Source: CAD feature listing. Evaluate the final solid. Frame: model axes, mm. Give positions to 0.01 mm unless a question says otherwise; leave off trailing zeros. Loops run counter-clockwise (first coordinate to the right, second up) from the corner with the lowest first, then second, coordinate; pieces in that order, holes last. Notation, with made-up numbers: (27, -37) -> (81, -37) arc R21 ccw to (81, -33) -> close; hole circle Ø7 at (53.25, 15). An arc over 180 degrees is marked (long way). Put each result on its own line as item: value.
```python
from build123d import *

# Parameters (mm, degrees)
ESBO_O1_W                  = 54
ESBO_O1_H                  = 15
RESSALTO_EXTRUS_O1_DEPTH   = 1.2
CORTE_EXTRUS_O1_DEPTH      = 5
CORTE_EXTRUS_O1_DEPTH_BACK = 1.2
ESBO_O2_R                  = 2


with BuildPart() as part:
    # Esboço1 → Ressalto-extrusão1 (new body)
    with BuildSketch(Plane.XY):
        Rectangle(ESBO_O1_W, ESBO_O1_H)
    extrude(amount=RESSALTO_EXTRUS_O1_DEPTH)

    # Esboço2 → Corte-extrusão1 (cut, two sides: drawn at the far end of the back side and taken through both)
    with BuildSketch(Plane.XY.offset(-CORTE_EXTRUS_O1_DEPTH_BACK)):
        with Locations(Location((-21.8, 0, 0), (0, 0, 180))):
            Circle(ESBO_O2_R)
        with Locations(Location((21.8, 0, 0), (0, 0, 180))):
            Circle(ESBO_O2_R)
    extrude(amount=CORTE_EXTRUS_O1_DEPTH + CORTE_EXTRUS_O1_DEPTH_BACK, mode=Mode.SUBTRACT)


solid = part.part
```
(1) Section C-C on z = 0.9. Return loops of the section in (x, y), then the cut area to 3 significant figures.
Calculated:
outline: (-27, -7.5) -> (27, -7.5) -> (27, 7.5) -> (-27, 7.5) -> close; hole circle Ø4 at (-21.8, 0); hole circle Ø4 at (21.8, 0)
area: 785 mm²
(2) Section A-A on x = 21.8. Return loops of the section in (y, z), then the cut area to 3 significant figures.
Calculated:
outline: (-7.5, 0) -> (-2, 0) -> (-2, 1.2) -> (-7.5, 1.2) -> close; (2, 0) -> (7.5, 0) -> (7.5, 1.2) -> (2, 1.2) -> close
area: 13.2 mm²
(3) Draft query along X for faces 1 (the flat face through (-27, 0, 1)), 2 (the flat face through (27, 0, 1)), 3 (the flat face through (0, 7.5, 1)), 4 (the cylindrical face through (-19.802, -0.088, 0.592)). Return one class per face: released by +X, released by -X, zero draft, split by the parting line, or undercut.
Calculated:
face 1: released by -X
face 2: released by +X
face 3: zero draft
face 4: undercut
(4) Line query: probe 1 along Y at (x, z) = (21.8, 0.65); probe 2 along X at (y, z) = (1.75, 0.3); probe 3 along Y at (x, z) = (-21, 1.1). Output: solid intervals per line, ascending. Write a range as from..to.
Calculated:
probe 1: y = -7.5..-2, 2..7.5
probe 2: x = -27..-22.77, -20.83..20.83, 22.77..27
probe 3: y = -7.5..-1.83, 1.83..7.5
(5) First-contact query: P1, Ø6.5, axis at x = 21.8, y = 0, coming from the +Z side. Flat tip, straight axial feed; report the tip coordinate or a pass-through.
Calculated:
P1: stops at z = 1.2
(6) Section B-B on y = 0. Return loops of the section in (x, z).
Calculated:
outline: (-27, 0) -> (-23.8, 0) -> (-23.8, 1.2) -> (-27, 1.2) -> close; (-19.8, 0) -> (19.8, 0) -> (19.8, 1.2) -> (-19.8, 1.2) -> close; (23.8, 0) -> (27, 0) -> (27, 1.2) -> (23.8, 1.2) -> close
